from build123d import *

# Parameters (mm, degrees)
F0_R     = 4.318
F1_DEPTH = 3.81
F2_DEPTH = 52.07
F4_DEPTH = 43.18
F6_DEPTH = 10.16
F7_R     = 2.54
F8_R     = 1.27


with BuildPart() as f1:
    # F0 (on Top) → F1 (new body)
    with BuildSketch(Plane.XY):
        with BuildLine():
            ThreePointArc((10.16, 5.08), (5.08, 5.08), (5.08, 10.16))
            ThreePointArc((5.08, 10.16), (0, 15.24), (-5.08, 10.16))
            ThreePointArc((-5.08, 10.16), (-5.08, 5.08), (-10.16, 5.08))
            ThreePointArc((-10.16, 5.08), (-15.24, 0), (-10.16, -5.08))
            ThreePointArc((-10.16, -5.08), (-5.08, -5.08), (-5.08, -10.16))
            ThreePointArc((-5.08, -10.16), (0, -15.24), (5.08, -10.16))
            ThreePointArc((5.08, -10.16), (5.08, -5.08), (10.16, -5.08))
            ThreePointArc((10.16, -5.08), (15.24, 0), (10.16, 5.08))
        make_face()
        Circle(F0_R, mode=Mode.SUBTRACT)
    extrude(amount=F1_DEPTH)

    # F0 (on Top) → F2 (join)
    with BuildSketch(Plane.XY):
        Circle(F0_R)
    extrude(amount=F2_DEPTH)

    # F3 (on face) → F4 (cut)
    with BuildSketch(Plane.XY.offset(52.07)):
        with BuildLine():
            Line((1.778, -3.9349510797), (1.778, 3.9349510797))
            ThreePointArc((1.778, 3.9349510797), (0, 4.318), (-1.778, 3.9349510797))
            Line((-1.778, 3.9349510797), (-1.778, -3.9349510797))
            ThreePointArc((-1.778, -3.9349510797), (0, -4.318), (1.778, -3.9349510797))
        make_face()
    extrude(amount=-F4_DEPTH, mode=Mode.SUBTRACT)

    # F5 (on face) → F6 (join)
    with BuildSketch(Plane.XY.offset(52.07)):
        with BuildLine():
            Line((1.778, -3.9349510797), (1.778, 3.9349510797))
            ThreePointArc((1.778, 3.9349510797), (-4.318, 0), (1.778, -3.9349510797))
        make_face()
        with BuildLine():
            ThreePointArc((1.778, -3.9349510797), (3.6278456417, -2.3417642922), (4.318, 0))
            ThreePointArc((4.318, 0), (3.6278456417, 2.3417642922), (1.778, 3.9349510797))
            Line((1.778, 3.9349510797), (1.778, -3.9349510797))
        make_face()
    extrude(amount=F6_DEPTH)

    # F7
    f7_edges = [f1.edges().sort_by_distance(p)[0] for p in [
        (-5.08, -10.16, 1.905),
        (-10.16, -5.08, 1.905),
        (5.08, -10.16, 1.905),
        (10.16, -5.08, 1.905),
        (10.16, 5.08, 1.905),
        (5.08, 10.16, 1.905),
        (-10.16, 5.08, 1.905),
        (-5.08, 10.16, 1.905),
    ]]
    fillet(f7_edges, radius=F7_R)

    # F8
    f8_edges = [f1.edges().sort_by_distance(p)[0] for p in [
        (-15.24, 0, 0),
        (-5.08, -5.08, 0),
        (0, -15.24, 0),
        (-10.547376, -4.949482, 0),
        (5.08, -5.08, 0),
        (4.949482, -10.547376, 0),
        (10.547376, -4.949482, 0),
        (15.24, 0, 0),
        (10.547376, 4.949482, 0),
        (5.08, 5.08, 0),
        (4.949482, 10.547376, 0),
        (0, 15.24, 0),
        (-4.949482, 10.547376, 0),
        (-5.08, 5.08, 0),
        (-10.547376, 4.949482, 0),
        (-4.949482, -10.547376, 0),
    ]]
    fillet(f8_edges, radius=F8_R)


solid = f1.part
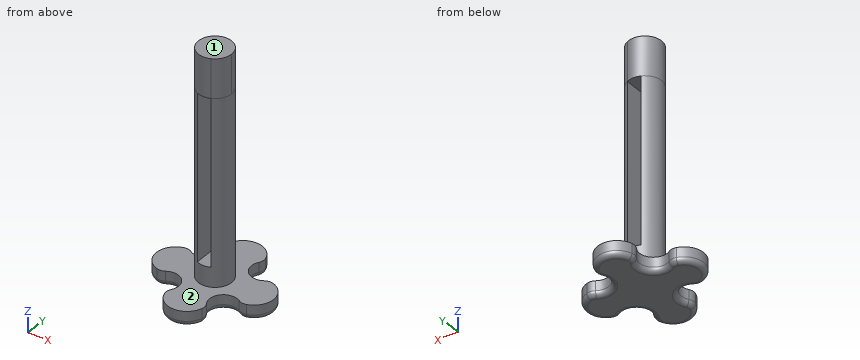
Verification items for the finished model (mm, model axes). Face numbers are marked on the shaded views. A direction names the side the tool comes from. Round coordinates to 2 decimals unless told otherwise and drop trailing zeros. Loops run counter-clockwise (first coordinate to the right, second up) from the corner with the lowest first, then second, coordinate; pieces in that order, holes last. Notation, with made-up numbers: (39, 59.25) - (62, 59.25) arc R22 ccw to (62, 98.25) - close; hole circle Ø3 at (-27.75, 70.5). An arc over 180 degrees is marked (long way). Answer in a Markdown table with one row per item. Add a question column.
Q1. Section check B-B on z = 47. Enter the section's corners in (x, y).
Q2. Gauge pin test, flat ends, axial feed: pin 1 (3 mm diameter, centred on x = 4, y = 11, fed in from +Z); pin 2 (1.5 mm diameter, centred on y = -5.5, z = 25.5, fed in from -X); pin 3 (6.5 mm diameter, centred on y = 0.5, z = 30.5, fed in from -X); pin 4 (8.5 mm diameter, centred on y = -1, z = 40.5, fed in from +X). Record the tip position at first contact, or that the pin passes through.
Q3. Section check A-A on x = 0. Enter the section's corners in (y, z), plus the area to 3 significant figures.
Q4. Material ranges on line 1 (Z direction, x = -2, y = 9); line 2 (Z direction, x = -1, y = -4); line 3 (X direction, y = -3, z = 59), recorded low to high.
Q5. Tool access check on the marked faces 1 and 2. Record the directions out of +Z, -Z, +X, -X, +Y, -Y that give a thin tool (end or side, any length) a straight path to the whole face; none if there is none.
Found:
| question | item | result |
|---|---|---|
| 1 | outline | (-1.78, -3.93) - (-1.78, 3.93) arc R4.32 ccw to start; (1.78, -3.93) arc R4.32 ccw to (1.78, 3.93) - close |
| 2 | pin 1 | stops at z = 3.81 |
| 2 | pin 2 | passes through |
| 2 | pin 3 | stops at x = -4.32 |
| 2 | pin 4 | stops at x = 4.32 |
| 3 | outline | (-15.24, 1.27) arc R1.27 ccw to (-13.97, 0) - (13.97, 0) arc R1.27 ccw to (15.24, 1.27) - (15.24, 3.81) - (4.32, 3.81) - (4.32, 8.89) - (-4.32, 8.89) - (-4.32, 3.81) - (-15.24, 3.81) - close; (-4.32, 52.07) - (4.32, 52.07) - (4.32, 62.23) - (-4.32, 62.23) - close |
| 3 | area | 247 mm² |
| 4 | line 1 | z = 0 to 3.81 |
| 4 | line 2 | z = 0 to 8.89, 52.07 to 62.23 |
| 4 | line 3 | x = -3.11 to 3.11 |
| 5 | face 1 | +Z, +X, -X, +Y, -Y |
| 5 | face 2 | +Z |
